The listing builds one solid part. Answer for the finished solid, in the listing's coordinates (mm). A direction names the side the tool comes from. Round coordinates to 2 decimals unless told otherwise and drop trailing zeros. Loops run counter-clockwise (first coordinate to the right, second up) from the corner with the lowest first, then second, coordinate; pieces in that order, holes last. Notation, with made-up numbers: (13.5, 51) - (17.5, 51) arc R37 cw to (17.5, 90) - close; hole circle Ø7 at (57.25, 6). An arc over 180 degrees is marked (long way). One line per item, written item: value.
Autodesk Inventor part; units mm, degrees
ref_plane "YZ Plane" through (0, 0, 0) normal (1, 0, 0) x (0, 1, 0)
ref_plane "XZ Plane" through (0, 0, 0) normal (0, 1, 0) x (-1, 0, 0)
ref_plane "XY Plane" through (0, 0, 0) normal (0, 0, 1) x (1, 0, 0)
sketch "Skizze1" plane through (0, 0, 0) normal (0, 1, 0) x (-1, 0, 0)
  line L0 (-92.5, -10) -> (92.5, -10)
  line L1 (92.5, -10) -> (92.5, 10)
  line L2 (92.5, 10) -> (-92.5, 10)
  line L3 (-92.5, 10) -> (-92.5, -10)
  line L4 (-92.5, -10) -> (92.5, 10) construction
  line L5 (92.5, -10) -> (-92.5, 10) construction
  point P0 (0, 0)
  dimension "d0" = 20
  dimension "d1" = 185
extrude "Extrusion1" add sketch "Skizze1" along normal blind 10
sketch "Skizze2" plane through (92.5, 0, 10) normal (1, 0, 0) x (0, 0, -1)
  line L0 (20, 10) -> (0, 10)
  line L1 (4, 10) -> (16, 10)
  line L2 (16, 10) -> (16, 4)
  line L3 (16, 4) -> (4, 4)
  line L4 (4, 4) -> (4, 10)
  line L5 (0, 0) -> (0, 10)
  line L6 (20, 0) -> (20, 10)
  line L7 (0, 0) -> (20, 0)
  point P0 (10, 0)
  point P1 (16, 7)
  point P2 (10, 4)
  dimension "d4" = 4
  dimension "d5" = 4
  dimension "d6" = 4
extrude "Extrusion2" cut sketch "Skizze2" against normal blind 181 contours L2 L3 L4 L0
sketch "Skizze3" plane through (0, 10, 0) normal (0, 1, 0) x (1, 0, 0)
  line L0 (-59.65, -9.75) -> (-40.05, -9.75)
  line L1 (-40.05, -9.75) -> (-40.05, -6.25)
  line L2 (-40.05, -6.25) -> (-59.65, -6.25)
  line L3 (-59.65, -6.25) -> (-59.65, -9.75)
  line L4 (-92.5, 10) -> (-92.5, -10)
  line L5 (92.5, -6) -> (-88.5, -6)
  line L6 (-59.65, 6.25) -> (-40, 6.25)
  line L7 (-40, 6.25) -> (-40, 9.75)
  line L8 (-40, 9.75) -> (-59.65, 9.75)
  line L9 (-59.65, 9.75) -> (-59.65, 6.25)
  line L10 (-88.5, 6) -> (92.5, 6)
  line L11 (40.05, -9.75) -> (59.65, -9.75)
  line L12 (59.65, -9.75) -> (59.65, -6.25)
  line L13 (59.65, -6.25) -> (40.05, -6.25)
  line L14 (40.05, -6.25) -> (40.05, -9.75)
  line L15 (92.5, -10) -> (92.5, -6)
  line L16 (40.0125, 6.25) -> (59.65, 6.25)
  line L17 (59.65, 6.25) -> (59.65, 9.75)
  line L18 (59.65, 9.75) -> (40.0125, 9.75)
  line L19 (40.0125, 9.75) -> (40.0125, 6.25)
  point P0 (0, 0)
  point P1 (-59.65, -8)
  point P2 (92.5, -8)
  point P3 (59.65, -8)
  dimension "d9" = 3.5
  dimension "d10" = 32.85
  dimension "d11" = 0.25
  dimension "d12" = 19.6
  dimension "d13" = 0.25
  dimension "d14" = 3.5
  dimension "d15" = 32.85
  dimension "d16" = 0.25
  dimension "d17" = 19.6
  dimension "d18" = 3.5
  dimension "d19" = 0.25
  dimension "d20" = 3.5
  dimension "d23" = 0
  dimension "d24" = 0
extrude "Extrusion3" add sketch "Skizze3" along normal blind 3.925
fillet "Rundung1" radius 1 26 edges at (-49.85, 13.925, 9.75) (-49.85, 13.925, 6.25) (-59.65, 13.925, 8) (-40.05, 13.925, 8) (-59.65, 13.925, -8) (-49.825, 13.925, -6.25) (-49.825, 13.925, -9.75) (-40, 13.925, -8) (40.0125, 13.925, -8) (49.8312, 13.925, -9.75) (49.8312, 13.925, -6.25) (59.65, 13.925, -8) (40.05, 13.925, 8) (49.85, 13.925, 9.75) (49.85, 13.925, 6.25) (59.65, 13.925, 8) (92.5, 5, 10) (92.5, 5, -10) (-92.5, 5, -10) (-92.5, 5, 10) (-92.5, 0, 0) (0, 0, 10) (0, 0, -10) (92.5, 0, 0) (2, 4, -6) (2, 4, 6)
properties part number "Kabelschacht 001"
1) For a pull along Z with two mould halves and no side action, classify faces 4 (the flat face through (-50, 11, -9.75)), 5 (the flat face through (-50, 11, 9.75)), 6 (the flat face through (-40.05, 11, 8)), 7 (the flat face through (50, 11, 6.25)) as released by +Z, released by -Z, zero draft, split by the parting line, or undercut.
Final values:
face 4: released by -Z
face 5: released by +Z
face 6: zero draft
face 7: undercut
2) A cutting plane is placed at A-A on x = -73.5. Give the vertices of the cut face in (y, z).
Final values:
outline: (0, -9) arc R1 ccw to (1, -10) - (10, -10) - (10, -6) - (5, -6) arc R1 cw to (4, -5) - (4, 5) arc R1 cw to (5, 6) - (10, 6) - (10, 10) - (1, 10) arc R1 ccw to (0, 9) - close
3) Consider L1, parallel to Z at x = -59.5, y = 7; L2, parallel to X at y = 10.5, z = -8.25; L3, parallel to Z at x = 50.5, y = 12.75. Determine where each line is inside the solid, lowest interval first.
Final values:
L1: -10 to -6, 6 to 10
L2: -59.65 to -40, 40.01 to 59.65
L3: -9.75 to -6.25, 6.25 to 9.75
4) A cutting plane is placed at D-D on x = -47. Give the vertices of the cut face in (y, z) (3 decimals), and give its area (3 significant figures).
Final values:
outline: (0, -9) arc R1 ccw to (1, -10) - (10, -10) - (10, -9.75) - (12.925, -9.75) arc R1 ccw to (13.925, -8.75) - (13.925, -7.25) arc R1 ccw to (12.925, -6.25) - (10, -6.25) - (10, -6) - (5, -6) arc R1 cw to (4, -5) - (4, 5) arc R1 cw to (5, 6) - (10, 6) - (10, 6.25) - (12.925, 6.25) arc R1 ccw to (13.925, 7.25) - (13.925, 8.75) arc R1 ccw to (12.925, 9.75) - (10, 9.75) - (10, 10) - (1, 10) arc R1 ccw to (0, 9) - close
area: 155 mm2
5) A cutting plane is placed at C-C on y = 6.5. Give the vertices of the cut face in (x, z).
Final values:
outline: (-92.5, -9) arc R1 ccw to (-91.5, -10) - (91.5, -10) arc R1 ccw to (92.5, -9) - (92.5, -6) - (-88.5, -6) - (-88.5, 6) - (92.5, 6) - (92.5, 9) arc R1 ccw to (91.5, 10) - (-91.5, 10) arc R1 ccw to (-92.5, 9) - close
6) Each of these flat-tipped pins is pushed along its axis until it touches: pin 1 Ø1.5 at (y, z) = (11.5, 8.5) entering from +X; pin 2 Ø1.5 at (y, z) = (12, -8) entering from -X; pin 3 Ø0.9 at (x, y) = (-50.5, 11) entering from -Z; pin 4 Ø2.5 at (y, z) = (11, 7.5) entering from -X. Where does it stop, or does it pass through?
Final values:
pin 1: x = 59.65
pin 2: x = -59.65
pin 3: z = -9.75
pin 4: x = -92.5
7) For faces 1 (the flat face through (3, 8, -6)), 2 (the flat face through (-59.65, 11, 8)), 3 (the flat face through (50, 11, 9.75)), determine the directions among +Z, -Z, +X, -X, +Y, -Y from which every point of the face is accessible in a straight line to the end or side of a thin tool.
Final values:
face 1: +X, +Y
face 2: +Z, -Z, -X, +Y
face 3: +Z, +X, -X, +Y
8) A cutting plane is placed at B-B on z = 3. Give the vertices of the cut face in (x, y).
Final values:
outline: (-92.5, 1) arc R1 ccw to (-91.5, 0) - (91.5, 0) arc R1 ccw to (92.5, 1) - (92.5, 4) - (-88.5, 4) - (-88.5, 10) - (-92.5, 10) - close
